Work out the finished part from the listing and answer in its coordinate system (mm). Coordinates: 2 decimals unless noted, no trailing zeros. Order: outer loops, then holes, each group sorted by start corner. A loop starts at its lowest first (then second) coordinate and runs counter-clockwise, first axis right, second up. Notation, with made-up numbers: M -0.5,32 L 8.5,32 A16 cw 8.5,41 Z; hole C -10,-16 d6. An arc over 180 degrees is marked long. Use a Markdown table: item, result.
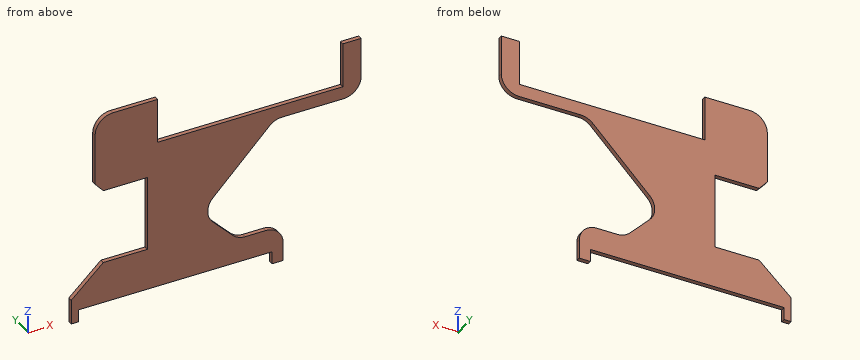
from build123d import *

# Parameters (mm, degrees)
BOSS_EXTRUDE1_DEPTH = 6.35


with BuildPart() as part:
    # Sketch2 → Boss-Extrude1 (new body)
    with BuildSketch(Plane(origin=(0, 0, 0), x_dir=(1, 0, 0), z_dir=(0, 1, 0))):
        with BuildLine():
            Line((-25.273, -79.248), (-25.273, -142.748))
            Line((-25.273, -142.748), (-89.721716587, -142.748))
            ThreePointArc((-89.721716587, -142.748), (-107.772031391, -135.271314803), (-115.248716587, -117.221))
            Line((-115.248716587, -117.221), (-115.248716587, -44.590319773))
            Line((-115.248716587, -44.590319773), (-103.51054261, -31.623))
            Line((-103.51054261, -31.623), (-40.0812, -31.623))
            Line((-40.0812, -31.623), (-40.0812, 0))
            Line((-40.0812, 0), (-40.0812, 74.803))
            Line((-40.0812, 74.803), (-103.503143824, 74.803))
            Line((-103.503143824, 74.803), (-149.633756095, 116.560985613))
            Line((-149.633756095, 116.560985613), (-149.633756095, 151.638))
            Line((-149.633756095, 151.638), (-139.573, 151.638))
            Line((-139.573, 151.638), (-139.573, 133.858))
            Line((-139.573, 133.858), (0, 133.858))
            Line((0, 133.858), (139.573, 133.858))
            Line((139.573, 133.858), (139.573, 151.638))
            Line((139.573, 151.638), (155.334898669, 151.638))
            Line((155.334898669, 151.638), (155.334898669, 125.037492411))
            ThreePointArc((155.334898669, 125.037492411), (147.858213472, 106.987177608), (129.807898669, 99.510492411))
            Line((129.807898669, 99.510492411), (100.730063349, 99.510492411))
            ThreePointArc((100.730063349, 99.510492411), (91.058504963, 97.586699836), (82.859353668, 92.108202092))
            Line((82.859353668, 92.108202092), (54.18030231, 63.429150734))
            ThreePointArc((54.18030231, 63.429150734), (46.778011991, 45.558441053), (54.18030231, 27.687731372))
            Line((54.18030231, 27.687731372), (135.638427829, -53.770394147))
            ThreePointArc((135.638427829, -53.770394147), (143.837579124, -59.248891891), (153.50913751, -61.172684466))
            Line((153.50913751, -61.172684466), (242.125928412, -61.172684466))
            ThreePointArc((242.125928412, -61.172684466), (260.176243215, -68.649369662), (267.652928412, -86.699684466))
            Line((267.652928412, -86.699684466), (267.652928412, -142.748))
            Line((267.652928412, -142.748), (241.173, -142.748))
            Line((241.173, -142.748), (241.173, -79.248))
            Line((241.173, -79.248), (0, -79.248))
            Line((0, -79.248), (-25.273, -79.248))
        make_face()
    extrude(amount=BOSS_EXTRUDE1_DEPTH)


solid = part.part
1. Find the intervals of material crossed by probe 1 along Z at (x, y) = (-63, 1); probe 2 along X at (y, z) = (1.5, 98.5); probe 3 along Z at (x, y) = (216.5, 1), in increasing order.
Answers below:
| item | result |
|---|---|
| probe 1 | -133.86 to -74.8, 31.62 to 142.75 |
| probe 2 | -115.25 to -25.27, 241.17 to 267.65 |
| probe 3 | 61.17 to 79.25 |
2. Section D-D on x = 171 is taken. Determine the outline of the cut face in (y, z), then the cut area to 3 significant figures.
Answers below:
| item | result |
|---|---|
| outline | M 0,61.17 L 6.35,61.17 L 6.35,79.25 L 0,79.25 Z |
| area | 115 mm² |
3. Section A-A on x = -58 is taken. Determine the outline of the cut face in (y, z).
Answers below:
| item | result |
|---|---|
| outline | M 0,-133.86 L 6.35,-133.86 L 6.35,-74.8 L 0,-74.8 Z; M 0,31.62 L 6.35,31.62 L 6.35,142.75 L 0,142.75 Z |
4. Section B-B on z = 101.5 is taken. Determine the outline of the cut face in (x, y), then the cut area to 3 significant figures.
Answers below:
| item | result |
|---|---|
| outline | M -115.25,0 L -25.27,0 L -25.27,6.35 L -115.25,6.35 Z; M 241.17,0 L 267.65,0 L 267.65,6.35 L 241.17,6.35 Z |
| area | 739 mm² |
5. Flat-ended cylindrical pins translate along their axes: P1, Ø1.5, axis at x = 102, y = 4, coming from the -Z side; P2, Ø1.9, axis at y = 4.5, z = 87.5, coming from the -X side; P3, Ø3, axis at y = 2, z = -145.5, coming from the +X side. Find the tip coordinate at first contact, or state that the pin passes through.
Answers below:
| item | result |
|---|---|
| P1 | z = -133.86 |
| P2 | x = -115.25 |
| P3 | x = 155.33 |
